from build123d import *

# Parameters (mm, degrees)
BOSS_EXTRUDE1_DEPTH          = 12.7
F_10_0_1935_DIAMETER_HOLE1_D = 4.9149


with BuildPart() as part:
    # Sketch1 → Boss-Extrude1 (new body)
    with BuildSketch(Plane.XY):
        with BuildLine():
            ThreePointArc((-38.262949069, 15.478125), (0, -41.275), (38.262949069, 15.478125))
            Line((38.262949069, 15.478125), (29.433037746, 37.30625))
            ThreePointArc((29.433037746, 37.30625), (0, 57.15), (-29.433037746, 37.30625))
            Line((-29.433037746, 37.30625), (-38.262949069, 15.478125))
        make_face()
    extrude(amount=BOSS_EXTRUDE1_DEPTH)

    # #10 (0.1935) Diameter Hole1 (through all)
    with Locations(Plane.XY.offset(12.7)):
        with Locations((0, 0)):
            Hole(F_10_0_1935_DIAMETER_HOLE1_D / 2)


solid = part.part
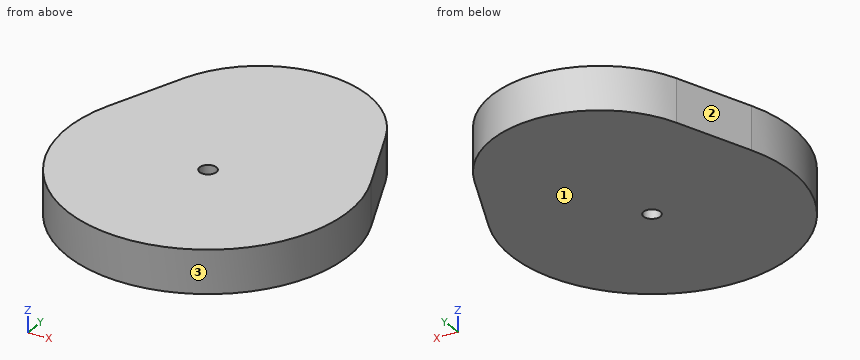
The listing builds one solid part. Answer for the finished solid, in the listing's coordinates (mm). Face numbers are marked on the shaded views. Give positions to 0.01 mm unless a question says otherwise; leave off trailing zeros. Order: outer loops, then holes, each group sorted by start corner. A loop starts at its lowest first (then second) coordinate and runs counter-clockwise, first axis right, second up. Notation, with made-up numbers: (51.5, 37.5) - (109.5, 37.5) arc R20 ccw to (109.5, 58.5) - close; hole circle Ø11 at (-34.75, 10.25). An arc over 180 degrees is marked (long way). One line per item, written item: value. Start each with the question number.
1) A cutting plane is placed at A-A on x = 0. Give the vertices of the cut face in (y, z) (3 decimals), then the cut area to 3 significant figures.
2) A cutting plane is placed at D-D on y = 24. Give the vertices of the cut face in (x, z), then the cut area to 3 significant figures.
3) The mould has two halves that part along X. Classify the marked faces 1, 2 and 3: released by +X, released by -X, zero draft, split by the parting line, or undercut.
4) A cutting plane is placed at C-C on z = 10. Give the vertices of the cut face in (x, y) (3 decimals), then the cut area to 3 significant figures.
5) Find the intervals of material crossed by L1, parallel to Y at x = 0, z = 4.75 (3 decimals); L2, parallel to X at y = 24, z = 4; L3, parallel to X at y = -19, z = 9.25, in increasing order.
6) Given pin 1 Ø1 at (x, z) = (-10.5, 6.5) entering from -Y; pin 2 Ø2 at (y, z) = (-22.5, 2.5) entering from +X; pin 3 Ø4 at (x, z) = (13, 4.5) entering from +Y; pin 4 Ø6 at (x, y) = (22.5, 38) entering from -Z, each flat-ended and moving along its own axis, determine where each tip first touches the part or whether it passes through.
7) A cutting plane is placed at B-B on y = 0. Give the vertices of the cut face in (x, z) (3 decimals).
Answer sheet:
1. outline: (-41.275, 0) - (-2.457, 0) - (-2.457, 12.7) - (-41.275, 12.7) - close; (2.457, 0) - (57.15, 0) - (57.15, 12.7) - (2.457, 12.7) - close
1. area: 1,190 mm2
2. outline: (-34.82, 0) - (34.82, 0) - (34.82, 12.7) - (-34.82, 12.7) - close
2. area: 884 mm2
3. face 1: zero draft
3. face 2: released by -X
3. face 3: split by the parting line
4. outline: (-38.263, 15.478) arc R41.275 ccw (long way) to (38.263, 15.478) - (29.433, 37.306) arc R31.75 ccw to (-29.433, 37.306) - close; hole circle Ø4.915 at (0, 0)
4. area: 6,230 mm2
5. L1: y = -41.275 to -2.457, 2.457 to 57.15
5. L2: x = -34.82 to 34.82
5. L3: x = -36.64 to 36.64
6. pin 1: stops at y = -40.05
6. pin 2: stops at x = 35.23
6. pin 3: stops at y = 55.18
6. pin 4: stops at z = 0
7. outline: (-41.275, 0) - (-2.457, 0) - (-2.457, 12.7) - (-41.275, 12.7) - close; (2.457, 0) - (41.275, 0) - (41.275, 12.7) - (2.457, 12.7) - close
